Can you work these out from the model? Positions are in its coordinate system, mm. A direction names the side the tool comes from. Give positions to 0.01 mm unless a question says otherwise; leave off trailing zeros. Write each loop counter-clockwise with the first axis right and the second up, starting at its lowest first coordinate (ties: lowest second). Pieces come first, ordered by that corner, then holes. Notation, with made-up numbers: (-36, 17.5) -> (20, 17.5) arc R23 ccw to (20, 41.5) -> close; hole circle Ø6 at (-33, 84). An arc over 180 degrees is marked (long way). One line per item, written item: value.
from build123d import *

# Parameters (mm, degrees)
SKETCH1_W           = 50
SKETCH1_H           = 20
BOSS_EXTRUDE1_DEPTH = 124
CUT_EXTRUDE1_REACH  = 128.89
SKETCH4_W           = 50
SKETCH4_H           = 42.5
BOSS_EXTRUDE2_DEPTH = 5
CUT_EXTRUDE2_DEPTH  = 3
SKETCH6_R           = 3.45
CUT_EXTRUDE3_DEPTH  = 134.834494571
SKETCH7_W           = 10
SKETCH7_H           = 10
CUT_EXTRUDE4_DEPTH  = 143.11702924
SKETCH8_R           = 3.05
CUT_EXTRUDE5_DEPTH  = 5
SKETCH9_R           = 3.15
CUT_EXTRUDE6_DEPTH  = 5


with BuildPart() as part:
    # Sketch1 → Boss-Extrude1 (new body)
    with BuildSketch(Plane.XY):
        Rectangle(SKETCH1_W, SKETCH1_H)
    extrude(amount=-BOSS_EXTRUDE1_DEPTH)

    # Sketch2 → Cut-Extrude1 (cut, up to next)
    with BuildSketch(Plane.XY, mode=Mode.PRIVATE) as cut_extrude1_sk1:
        Polygon((-10.499848989, 10.238924494), (0, 10.238924494), (10.499848989, 10.238924494), (10.499848989, 7.382817713), (9.707031275, 6.59), (3.792817713, 6.59), (3.292893219, 7.089924494), (-3.292893219, 7.089924494), (-3.792817713, 6.59), (-9.707031275, 6.59), (-10.499848989, 7.382817713), align=None)
    cut_extrude1_tool1 = extrude(cut_extrude1_sk1.sketch, amount=-CUT_EXTRUDE1_REACH, mode=Mode.PRIVATE) & part.part
    add(cut_extrude1_tool1.solids().sort_by_distance((0, 8.505261, 0))[0], mode=Mode.SUBTRACT)

    # Sketch4 → Boss-Extrude2 (add)
    with BuildSketch(Plane(origin=(0, 0, -124), x_dir=(-1, 0, 0), z_dir=(0, 0, -1))):
        with Locations((0, 11.25)):
            Rectangle(SKETCH4_W, SKETCH4_H)
    extrude(amount=BOSS_EXTRUDE2_DEPTH)

    # Sketch5 → Cut-Extrude2 (cut)
    with BuildSketch(Plane.XY.offset(-124)):
        with BuildLine():
            Line((-3.292893219, 7.089924494), (3.292893219, 7.089924494))
            Line((3.292893219, 7.089924494), (3.792817713, 6.59))
            Line((3.792817713, 6.59), (9.707031275, 6.59))
            Line((9.707031275, 6.59), (10.499848989, 7.382817713))
            Line((10.499848989, 7.382817713), (10.499848989, 9.99920802))
            Line((10.499848989, 9.99920802), (5.426401458, 13.551674225))
            ThreePointArc((5.426401458, 13.551674225), (5.112967061, 13.909077656), (4.999977894, 14.37082627))
            Line((4.999977894, 14.37082627), (4.999977894, 16.58982627))
            ThreePointArc((4.999977894, 16.58982627), (5.292871113, 17.296933051), (5.999977894, 17.58982627))
            Line((5.999977894, 17.58982627), (15.207084675, 17.58982627))
            Line((15.207084675, 17.58982627), (15.999902388, 18.382643983))
            Line((15.999902388, 18.382643983), (15.999902388, 25.796857545))
            Line((15.999902388, 25.796857545), (15.207084675, 26.589675258))
            Line((15.207084675, 26.589675258), (7.165888575, 26.589675258))
            Line((7.165888575, 26.589675258), (6.544410681, 25.089294897))
            Line((6.544410681, 25.089294897), (-6.544410681, 25.089294897))
            Line((-6.544410681, 25.089294897), (-7.165888575, 26.589675258))
            Line((-7.165888575, 26.589675258), (-15.207084675, 26.589675258))
            Line((-15.207084675, 26.589675258), (-15.999902388, 25.796857545))
            Line((-15.999902388, 25.796857545), (-15.999902388, 18.382643983))
            Line((-15.999902388, 18.382643983), (-15.207084675, 17.58982627))
            Line((-15.207084675, 17.58982627), (-5.999977894, 17.58982627))
            ThreePointArc((-5.999977894, 17.58982627), (-5.292871113, 17.296933051), (-4.999977894, 16.58982627))
            Line((-4.999977894, 16.58982627), (-4.999977894, 14.37082627))
            ThreePointArc((-4.999977894, 14.37082627), (-5.112967061, 13.909077656), (-5.426401458, 13.551674225))
            Line((-5.426401458, 13.551674225), (-10.499848989, 9.99920802))
            Line((-10.499848989, 9.99920802), (-10.499848989, 7.382817713))
            Line((-10.499848989, 7.382817713), (-9.707031275, 6.59))
            Line((-9.707031275, 6.59), (-3.792817713, 6.59))
            Line((-3.792817713, 6.59), (-3.292893219, 7.089924494))
        make_face()
    extrude(amount=-CUT_EXTRUDE2_DEPTH, mode=Mode.SUBTRACT)

    # Sketch6 → Cut-Extrude3 (cut, through all)
    with BuildSketch(Plane(origin=(0, 7.089924494, 0), x_dir=(1, 0, 0), z_dir=(0, 1, 0))):
        with Locations(Location((0, 92, 0), (0, 0, 270))):
            Circle(SKETCH6_R)
        with Locations(Location((0, 32, 0), (0, 0, 270))):
            Circle(SKETCH6_R)
    extrude(amount=-CUT_EXTRUDE3_DEPTH, mode=Mode.SUBTRACT)

    # Sketch7 → Cut-Extrude4 (cut, through all)
    with BuildSketch(Plane(origin=(25, 0, 0), x_dir=(0, 0, -1), z_dir=(1, 0, 0))):
        with Locations((124, -5)):
            Rectangle(SKETCH7_W, SKETCH7_H)
    extrude(amount=-CUT_EXTRUDE4_DEPTH, mode=Mode.SUBTRACT)

    # Sketch8 → Cut-Extrude5 (cut)
    with BuildSketch(Plane(origin=(25, 0, 0), x_dir=(0, 0, -1), z_dir=(1, 0, 0))):
        with Locations(Location((109, 0, 0), (0, 0, 90))):
            Circle(SKETCH8_R)
        with Locations(Location((65, 0, 0), (0, 0, 90))):
            Circle(SKETCH8_R)
    cut_extrude5 = extrude(amount=-CUT_EXTRUDE5_DEPTH, mode=Mode.SUBTRACT)

    # Mirror1: Cut-Extrude5 across plane
    add(cut_extrude5.mirror(Plane(origin=(0, 0, 0), x_dir=(0, 0, 1), z_dir=(1, 0, 0))), mode=Mode.SUBTRACT)

    # Sketch9 → Cut-Extrude6 (cut)
    with BuildSketch(Plane.XY):
        with Locations((-15, 0)):
            Circle(SKETCH9_R)
        with Locations((15, 0)):
            Circle(SKETCH9_R)
    extrude(amount=-CUT_EXTRUDE6_DEPTH, mode=Mode.SUBTRACT)


solid = part.part
1) If we section it at A-A (x = 0): Write out the boundary of the cut face in (y, z).
Answer list:
outline: (-10, -119) -> (0, -119) -> (0, -129) -> (32.5, -129) -> (32.5, -124) -> (25.09, -124) -> (25.09, -127) -> (7.09, -127) -> (7.09, -95.45) -> (-10, -95.45) -> close; (-10, -88.55) -> (7.09, -88.55) -> (7.09, -35.45) -> (-10, -35.45) -> close; (-10, -28.55) -> (7.09, -28.55) -> (7.09, 0) -> (-10, 0) -> close
2) If we section it at B-B (z = -22): Write out the boundary of the cut face in (x, y), and give its area (3 significant figures).
Answer list:
outline: (-25, -10) -> (25, -10) -> (25, 10) -> (10.5, 10) -> (10.5, 7.38) -> (9.71, 6.59) -> (3.79, 6.59) -> (3.29, 7.09) -> (-3.29, 7.09) -> (-3.79, 6.59) -> (-9.71, 6.59) -> (-10.5, 7.38) -> (-10.5, 10) -> (-25, 10) -> close
area: 933 mm^2
3) For faces 4 (the face through (0, 7.09, -15)), 5 (the face through (0, -5, -119)), 6 (the face through (22.535, -0.397, -105.976)), 7 (the face through (-18, 10, -61)), 8 (the face through (11.853, 0.138, -2.465)), which set-ups out of +Z, -Z, +X, -X, +Y, -Y let a thin tool reach every point of the face, with its end or its side?
Answer list:
face 4: +Z, +Y
face 5: -Z, +X, -X, -Y
face 6: +X
face 7: +Z, +X, -X, +Y
face 8: +Z
4) Will these pins go through, and if not, where does the flat tip stop? pin 1 (3 mm diameter, centred on x = 16, y = 1, fed in from +Z); pin 2 (5.5 mm diameter, centred on x = 0, z = -108.5, fed in from +Y); pin 3 (7.5 mm diameter, centred on x = -14.5, z = -43.5, fed in from +Y).
Answer list:
pin 1: stops at z = -5
pin 2: stops at y = 7.09
pin 3: stops at y = 10
5) We'd pull the mould along X, two halves only. Please class faces 1 (the face through (10.5, 9, -63)), 2 (the face through (20, 0, -109)), 3 (the face through (-22.535, -0.661, -67.977)): released by +X, released by -X, zero draft, split by the parting line, or undercut.
Answer list:
face 1: undercut
face 2: released by +X
face 3: zero draft
6) I need wall thicknesses on L1, parallel to Z at x = 0, y = 3.5; L2, parallel to Z at x = 0, y = -0.5; L3, parallel to X at y = -1.75, z = -32. Which ranges of each line are inside material? Lowest first, please.
Answer list:
L1: z = -129 to -95.45, -88.55 to -35.45, -28.55 to 0
L2: z = -119 to -95.45, -88.55 to -35.45, -28.55 to 0
L3: x = -25 to -3.45, 3.45 to 25
7) If we section it at C-C (y = 30.5): Write out the boundary of the cut face in (x, z).
Answer list:
outline: (-25, -129) -> (25, -129) -> (25, -124) -> (-25, -124) -> close
8) If we section it at D-D (z = -65): Write out the boundary of the cut face in (x, y), and give its area (3 significant figures).
Answer list:
outline: (-25, -10) -> (25, -10) -> (25, -3.05) -> (20, -3.05) -> (20, 3.05) -> (25, 3.05) -> (25, 10) -> (10.5, 10) -> (10.5, 7.38) -> (9.71, 6.59) -> (3.79, 6.59) -> (3.29, 7.09) -> (-3.29, 7.09) -> (-3.79, 6.59) -> (-9.71, 6.59) -> (-10.5, 7.38) -> (-10.5, 10) -> (-25, 10) -> (-25, 3.05) -> (-20, 3.05) -> (-20, -3.05) -> (-25, -3.05) -> close
area: 872 mm^2
